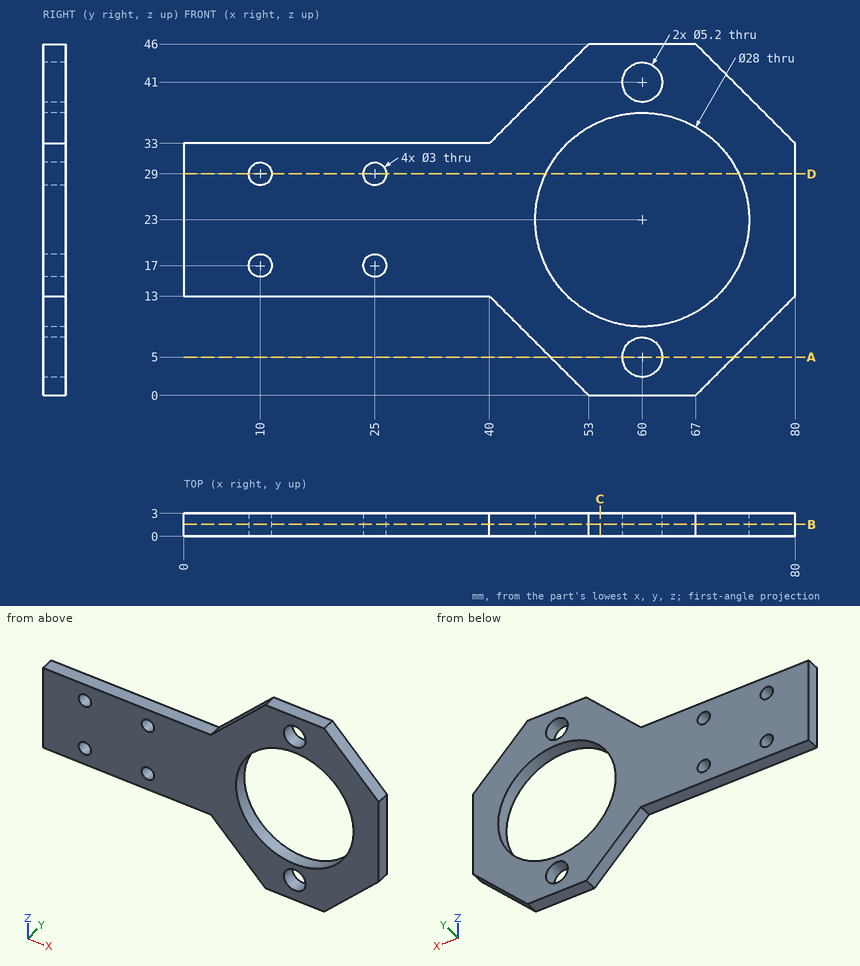
The drawing under review shows one solid part. Ordinate dimensions are in mm from its lowest x, y, z. Coordinates: 2 decimals unless noted, no trailing zeros. Order: outer loops, then holes, each group sorted by start corner. A loop starts at its lowest first (then second) coordinate and runs counter-clockwise, first axis right, second up. Notation, with made-up numbers: M 45,-12 L 104,-12 A21 cw 104,23 Z; hole C -23,62.25 d8. An arc over 180 degrees is marked long. One line per question, with ' | ' between items.
(1) For probe 1 along Z at (x, y) = (60, 2.25); probe 2 along X at (y, z) = (2.15, 17); probe 3 along X at (y, z) = (0.8, 23), list the stretches that pass through material, from the lowest coordinate up. Write a range as from..to.
Geometry results:
probe 1: z = 0..2.4, 7.6..9, 37..38.4, 43.6..46 | probe 2: x = 0..8.5, 11.5..23.5, 26.5..47.35, 72.65..80 | probe 3: x = 0..46, 74..80
(2) Add section C-C, the plane x = 54.5. Write out the cut boundary in (y, z), then the cut area to 3 significant figures.
Geometry results:
outline: M 0,0 L 3,0 L 3,10.13 L 0,10.13 Z; M 0,35.87 L 3,35.87 L 3,46 L 0,46 Z | area: 60.8 mm²
(3) Add section A-A, the plane z = 5. Write out the cut boundary in (x, y).
Geometry results:
outline: M 48,0 L 57.4,0 L 57.4,3 L 48,3 Z; M 62.6,0 L 72,0 L 72,3 L 62.6,3 Z
(4) Add section D-D, the plane z = 29. Write out the cut boundary in (x, y).
Geometry results:
outline: M 0,0 L 8.5,0 L 8.5,3 L 0,3 Z; M 11.5,0 L 23.5,0 L 23.5,3 L 11.5,3 Z; M 26.5,0 L 47.35,0 L 47.35,3 L 26.5,3 Z; M 72.65,0 L 80,0 L 80,3 L 72.65,3 Z
(5) Insertion check: pin 1 (1.8 mm diameter, centred on x = 25, z = 17, fed in from -Y); pin 2 (1.5 mm diameter, centred on y = 1.5, z = 7, fed in from +X). Each pin has a flat end and moves straight along its axis. Give the tip position at first contact, or say it passes through.
Geometry results:
pin 1: passes through | pin 2: stops at x = 74.75
(6) Add section B-B, the plane y = 1.55. Write out the cut boundary in (x, z).
Geometry results:
outline: M 0,13 L 40,13 L 53,0 L 67,0 L 80,13 L 80,33 L 67,46 L 53,46 L 40,33 L 0,33 Z; hole C 10,17 d3; hole C 10,29 d3; hole C 25,17 d3; hole C 25,29 d3; hole C 60,23 d28; hole C 60,5 d5.2; hole C 60,41 d5.2
